Autodesk Inventor part; units mm, degrees
ref_plane "Start Plane" through (0, 0, -18.5858) normal (0, 0, 1) x (1, 0, 0)
ref_plane "End Plane" through (0, 0, 1018.5858) normal (0, 0, 1) x (1, 0, 0)
ref_plane "Work Plane5" through (-20.7071, 0, -19.2929) normal (0.7071, 0, -0.7071) x (-0.7071, 0, -0.7071)
ref_plane "Start Plane" through (0, 0, -18.5858) normal (0, 0, 1) x (1, 0, 0)
ref_plane "End Plane" through (0, 0, 1018.5858) normal (0, 0, 1) x (1, 0, 0)
sketch "Sketch" plane through (0, 0, 0) normal (0, 0, 1) x (1, 0, 0)
  line L0 (-20, -15.5) -> (-20, 15.5)
  line L1 (-15.5, 20) -> (15.5, 20)
  line L2 (20, 15.5) -> (20, -15.5)
  line L3 (15.5, -20) -> (-15.5, -20)
  arc A0 (-20, -15.5) -> (-15.5, -20) centre (-15.5, -15.5) ccw
  arc A1 (-15.5, 20) -> (-20, 15.5) centre (-15.5, 15.5) ccw
  arc A2 (20, 15.5) -> (15.5, 20) centre (15.5, 15.5) ccw
  arc A3 (15.5, -20) -> (20, -15.5) centre (15.5, -15.5) ccw
  arc A4 (-15.5, 17) -> (-17, 15.5) centre (-15.5, 15.5) ccw
  line L4 (-15.5, 17) -> (15.5, 17)
  arc A5 (17, 15.5) -> (15.5, 17) centre (15.5, 15.5) ccw
  line L5 (17, 15.5) -> (17, -15.5)
  arc A6 (15.5, -17) -> (17, -15.5) centre (15.5, -15.5) ccw
  line L6 (15.5, -17) -> (-15.5, -17)
  arc A7 (-17, -15.5) -> (-15.5, -17) centre (-15.5, -15.5) ccw
  line L7 (-17, -15.5) -> (-17, 15.5)
  line L8 (0, 29.3048) -> (0, -29.3048) construction
  line L9 (-29.3048, 0) -> (29.3048, 0) construction
  dimension "d7" = 4.5
  dimension "d10" = 40
  dimension "d11" = 40
  dimension "d12" = 3
  dimension "d15" = 20
  dimension "d16" = 20
extrude "Body" add sketch "Sketch" along normal up to surface (1037.1716 mm away) from surface at -18.5858
sketch "Sketch3" plane through (0, 0, 0) normal (0, 0, 1) x (1, 0, 0)
  line L0 (0, 0) -> (10, 0)
ref_plane "Work Plane3" through (0, 0, 0) normal (0, -1, 0) x (1, 0, 0)
ref_plane "Work Plane5" through (-20.7071, 0, -19.2929) normal (0.7071, 0, -0.7071) x (-0.7071, 0, -0.7071)
split "Split2" plane through (-20.7071, 0, -19.2929) removes the side toward (0.7071, 0, -0.7071)
ref_plane "Work Plane8" through (-20.7071, 0, 1019.2929) normal (0.7071, 0, 0.7071) x (0.7071, 0, -0.7071)
split "Split5" plane through (-20.7071, 0, 1019.2929) removes the side toward (0.7071, 0, 0.7071)
sketch "Sketch4" plane through (0, 0, 0) normal (0, -1, 0) x (1, 0, 0)
  line L0 (-2, -18.5858) -> (12, -18.5858)
  line L1 (-2, 1018.5858) -> (12, 1018.5858)
  dimension "d18" = 1037.1716
equation "\"d7\" = G_IR"
equation "\"d10\" = G_H"
equation "\"d11\" = G_W"
equation "\"d12\" = G_T"
equation "\"d15\" = 0.5 * d10"
equation "\"d16\" = 0.5 * d11"
equation "\"d3\" = G_L"
equation "\"G_W\" = 40"
equation "\"G_H\" = 40"
equation "\"G_T\" = 3"
equation "\"G_IR\" = 4.5"
equation "\"G_L\" = d18"
equation "\"G_OFFSET_START\" = 18.58579"
equation "\"G_OFFSET_END\" = 18.58579"
equation "\"d13\" = -G_OFFSET_START"
equation "\"d14\" = G_OFFSET_END + B_L"
properties part number "ISO 12633-2 - 40x40x3 - 1037,17" material "Steel, Mild"
Could you check a few things on this model? Use its own coordinates, in mm. A direction names the side the tool comes from. Round coordinates to 2 decimals unless told otherwise and drop trailing zeros. Loops run counter-clockwise (first coordinate to the right, second up) from the corner with the lowest first, then second, coordinate; pieces in that order, holes last.
Q1. I want a section at B-B (x = 0). Write out the boundary of the cut face in (y, z).
Q2. For P1, Ø10, axis at x = -11.5, y = 15, coming from the +Z side; P2, Ø3, axis at x = -14.5, y = 4, coming from the +Z side (3 decimals), each with a flat end and sliding along its axis, tell me the tip position at first contact or that it passes through.
Q3. Thinking about a two-plate mould opening in X: for faces 1 (the flat face through (-20, 0, 493)), 2 (the flat face through (20, 0, 493)), 3 (the flat face through (17, 0, 493)), which applies, pulls with the +X half, pulls with the -X half, needs draft (parallel to the pull), parting line crosses it, or undercut?
Q4. On a 3-axis mill with a long thin cutter (end or side, diameter ignored), from which of +Z, -Z, +X, -X, +Y, -Y can I reach the whole of each face in a straight line? I mean faces 4 (the flat face through (-17, 0, 493)), 5 (the flat face through (-0.28, 18.058, 1.134)). Say none if no direction works.
Q5. I want a section at C-C (z = 762). Write out the boundary of the cut face in (x, y).
Q6. Please list where these lines run through material, in increasing order: L1, parallel to X at y = -12, z = 396; L2, parallel to Y at x = 18, z = 311.
Q7. I want a section at A-A (y = 3.5). Write out the boundary of the cut face in (x, z).
Answer below:
1. outline: (-20, 1.41) - (-17, 1.41) - (-17, 998.59) - (-20, 998.59) - close; (17, 1.41) - (20, 1.41) - (20, 998.59) - (17, 998.59) - close
2. P1: stops at z = 1014.73
2. P2: passes through
3. face 1: pulls with the -X half
3. face 2: pulls with the +X half
3. face 3: undercut
4. face 4: +Z, -Z
4. face 5: -Z, +X, +Y, -Y
5. outline: (-20, -15.5) arc R4.5 ccw to (-15.5, -20) - (15.5, -20) arc R4.5 ccw to (20, -15.5) - (20, 15.5) arc R4.5 ccw to (15.5, 20) - (-15.5, 20) arc R4.5 ccw to (-20, 15.5) - close; hole (-17, -15.5) arc R1.5 ccw to (-15.5, -17) - (15.5, -17) arc R1.5 ccw to (17, -15.5) - (17, 15.5) arc R1.5 ccw to (15.5, 17) - (-15.5, 17) arc R1.5 ccw to (-17, 15.5) - close
6. L1: x = -20 to -17, 17 to 20
6. L2: y = -19.24 to 19.24
7. outline: (-20, -18.59) - (-17, -15.59) - (-17, 1015.59) - (-20, 1018.59) - close; (17, 18.41) - (20, 21.41) - (20, 978.59) - (17, 981.59) - close
